Could you check a few things on this model? Use its own coordinates, in mm. Face numbers are marked on the shaded views. A direction names the side the tool comes from. Round coordinates to 2 decimals unless told otherwise and drop trailing zeros. Loops run counter-clockwise (first coordinate to the right, second up) from the corner with the lowest first, then second, coordinate; pieces in that order, holes last. Notation, with made-up numbers: M 64.5,2.5 L 113.5,2.5 A15 cw 113.5,11.5 Z; hole C 42.5,78.5 d4. An arc over 180 degrees is marked long. Return JSON: item names as keys, results as strings. Group by question number.
```python
from build123d import *

# Parameters (mm, degrees)
BOSS_EXTRU_1_DEPTH = 25
BOSS_EXTRU_4_START = 15
BOSS_EXTRU_4_DEPTH = 10
BOSS_EXTRU_5_START = -15
BOSS_EXTRU_5_DEPTH = 10
ESQUISSE1_9_W      = 15
ESQUISSE1_9_H      = 5
CONG_1_R           = 2


with BuildPart() as part:
    # Esquisse1 → Boss.-Extru.1 (new body, symmetric)
    with BuildSketch(Plane.XY):
        Polygon((10, 10), (0, 0), (100, 0), (90, 10), (90, 20), (20, 20), (20, 45), (10, 45), align=None)
    extrude(amount=BOSS_EXTRU_1_DEPTH, both=True)

    # Esquisse1_5 → Boss.-Extru.4 (add)
    with BuildSketch(Plane.XY.offset(BOSS_EXTRU_4_START)):
        Polygon((20, 45), (20, 20), (50, 20), align=None)
    extrude(amount=BOSS_EXTRU_4_DEPTH)

    # Esquisse1_6 → Boss.-Extru.5 (add)
    with BuildSketch(Plane.XY.offset(BOSS_EXTRU_5_START)):
        Polygon((20, 45), (20, 20), (50, 20), align=None)
        Polygon((50, 45), (20, 45), (50, 20), align=None)
    extrude(amount=-BOSS_EXTRU_5_DEPTH)

    # Esquisse1_9 → R_volution1 (revolve)
    with BuildSketch(Plane.XY):
        with Locations((72.5, 22.5)):
            Rectangle(ESQUISSE1_9_W, ESQUISSE1_9_H)
    revolve(axis=Axis((65, 46.334519573, 0), (0, -1, 0)))

    # Cong_1
    cong_1_edges = [part.edges().sort_by_distance(p)[0] for p in [
        (50, 20, 0),
    ]]
    fillet(cong_1_edges, radius=CONG_1_R)


solid = part.part
```
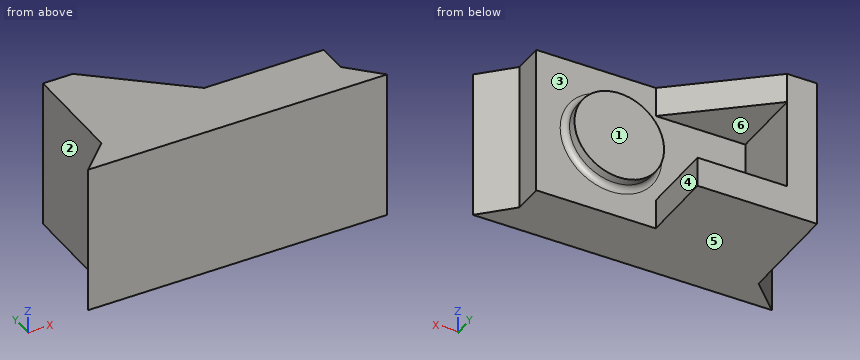
1. We'd pull the mould along Z, two halves only. Please class the marked faces 4, 5 and 6: +Z half, -Z half, draft (parallel to the pull), parting line (faces both ways), or undercut.
2. If we section it at D-D, the plane x = 65: Please give me the cut outline in (y, z).
3. If we section it at C-C, the plane z = 0: Please give me the cut outline in (x, y), then the cut area to 3 significant figures.
4. I'm going to push flat-ended pins straight in: pin 1 Ø10.5 at (y, z) = (27, -5) entering from -X; pin 2 Ø4 at (y, z) = (24, -9.5) entering from +X; pin 3 Ø11 at (y, z) = (13.5, -12.5) entering from +X. Where does each tip first touch, or does it pass through?
5. On a 3-axis mill with a long thin cutter (end or side, diameter ignored), from which of +Z, -Z, +X, -X, +Y, -Y can I reach the whole of each face in a straight line? I mean the marked faces 1, 2 and 3. Say none if no direction works.
6. I need wall thicknesses on probe 1 along X at (y, z) = (35, 14.5); probe 2 along Y at (x, z) = (21, -4); probe 3 along Z at (x, y) = (35.5, 36.5). Which ranges of each line are inside material? Lowest first, please.
7. If we section it at B-B, the plane x = 35: Please give me the cut outline in (y, z).
8. If we section it at A-A, the plane y = 26.5: Please give me the cut outline in (x, z), then the cut area to 3 significant figures.
Geometry results:
{
 "1": {"face 4": "draft", "face 5": "-Z half", "face 6": "undercut"},
 "2": {"outline": "M 0,-25 L 20,-25 L 20,-17 A2 cw 22,-15 L 25,-15 L 25,15 L 22,15 A2 cw 20,17 L 20,25 L 0,25 Z"},
 "3": {"outline": "M 0,0 L 100,0 L 90,10 L 90,20 L 82,20 A2 cw 80,22 L 80,25 L 50,25 L 50,22 A2 cw 48,20 L 20,20 L 20,45 L 10,45 L 10,10 Z", "area": "2,100 mm^2"},
 "4": {"pin 1": "x = 10", "pin 2": "x = 77.99", "pin 3": "x = 92"},
 "5": {"face 1": "+Z, -Z, +X, +Y", "face 2": "+Z, -Z, -X, +Y", "face 3": "+Y"},
 "6": {"probe 1": "10 to 20", "probe 2": "0 to 20", "probe 3": "-25 to -15"},
 "7": {"outline": "M 0,-25 L 45,-25 L 45,-15 L 20,-15 L 20,15 L 32.5,15 L 32.5,25 L 0,25 Z"},
 "8": {"outline": "M 10,-25 L 50,-25 L 50,-15 L 20,-15 L 20,15 L 42.2,15 L 42.2,25 L 10,25 Z", "area": "1,020 mm^2"}
}
